Input: part model. Units: mm. Frame: model coordinates. Coordinates: 2 decimals unless noted, no trailing zeros. Loops run counter-clockwise (first coordinate to the right, second up) from the corner with the lowest first, then second, coordinate; pieces in that order, holes last.
(1) Line query: L1, parallel to Z at x = 31.75, y = 3.6; L2, parallel to X at y = 1.65, z = 15; L3, parallel to X at y = 1.8, z = 0. Output: solid intervals per line, ascending.
(2) Section D-D, the plane z = 0. Return loops of the section in (x, y).
(3) Section B-B, the plane x = -31.75. Return loops of the section in (y, z), then the cut area to 4 significant figures.
(4) Section C-C, the plane y = 2.85. Give the number of separate pieces and of enclosed holes in the cut face, then the cut area to 3 significant figures.
(5) Section A-A, the plane z = -15. Return loops of the section in (x, y).
Autodesk Fusion 360 part; units mm, degrees
sketch "Sketch1" plane through (0, 0, 0) normal (0, 1, 0) x (1, 0, 0)
  line L0 (-20.75, -20) -> (20.75, -20) construction
  line L1 (20.75, -20) -> (20.75, 20) construction
  line L2 (20.75, 20) -> (-20.75, 20) construction
  line L3 (-20.75, 20) -> (-20.75, -20) construction
  line L4 (-20.75, -20) -> (20.75, 20) construction
  line L5 (20.75, -20) -> (-20.75, 20) construction
  circle A0 centre (-31.75, 0) radius 4.05
  circle A1 centre (31.75, 0) radius 4.05
  line L6 (25.5, 0) -> (-25.5, 0)
  line L7 (22.803, -2.697) -> (-22.803, -2.697)
  line L8 (-22.803, -2.697) -> (-22.803, -37.303)
  line L9 (-22.803, -37.303) -> (22.803, -37.303)
  line L10 (22.803, -37.303) -> (22.803, -2.697)
  line L11 (22.803, -2.697) -> (-22.803, -37.303) construction
  line L12 (-22.803, -2.697) -> (22.803, -37.303) construction
  line L13 (22.803, 2.697) -> (-22.803, 2.697)
  line L14 (-22.803, 2.697) -> (-22.803, 37.303)
  line L15 (-22.803, 37.303) -> (22.803, 37.303)
  line L16 (22.803, 37.303) -> (22.803, 2.697)
  line L17 (22.803, 2.697) -> (-22.803, 37.303) construction
  line L18 (-22.803, 2.697) -> (22.803, 37.303) construction
  circle A2 centre (-22.803, -37.303) radius 1.55
  circle A3 centre (22.803, -2.697) radius 1.55
  circle A4 centre (-22.803, 2.697) radius 1.55
  circle A5 centre (22.803, 37.303) radius 1.55
  circle A6 centre (-31.75, -15) radius 1.55
  circle A7 centre (-31.75, 15) radius 1.55
  circle A8 centre (31.75, -15) radius 1.55
  circle A9 centre (31.75, 15) radius 1.55
  line L19 (-47, -40) -> (47, -40)
  line L20 (47, -40) -> (47, 40)
  line L21 (47, 40) -> (-47, 40)
  line L22 (-47, 40) -> (-47, -40)
  line L23 (-47, -40) -> (47, 40) construction
  line L24 (47, -40) -> (-47, 40) construction
  point P0 (0, -20)
  point P1 (0, 20)
  point P2 (0, -20)
  point P3 (0, 20)
  dimension "d1" = 41.5
  dimension "d2" = 40
  dimension "d3" = 8.1
  dimension "d4" = 8.1
  dimension "d5" = 11
  dimension "d6" = 11
  dimension "d7" = 51
  dimension "d8" = 20
  dimension "d9" = 20
  dimension "d10" = 45.606
  dimension "d11" = 34.606
  dimension "d12" = 45.606
  dimension "d13" = 34.606
  dimension "d14" = 3.1
  dimension "d15" = 3.1
  dimension "d16" = 3.1
  dimension "d17" = 3.1
  dimension "d18" = 3.1
  dimension "d19" = 3.1
  dimension "d20" = 3.1
  dimension "d21" = 3.1
  dimension "d22" = 15
  dimension "d23" = 15
  dimension "d24" = 15
  dimension "d25" = 15
  dimension "d26" = 94
  dimension "d27" = 80
extrude "Extrude1" add sketch "Sketch1" along normal blind 5 contours L7 L8 L9 L10 A2 A3 | L13 L14 L15 L16 A4 A5 | L19 L20 L21 L22
fillet "Fillet1" radius 10 4 edges at (47, 2.5, 40) (47, 2.5, -40) (-47, 2.5, 40) (-47, 2.5, -40)
equation "d6 = d5"
equation "d23 = d22"
equation "d24 = d23"
equation "d25 = d22"
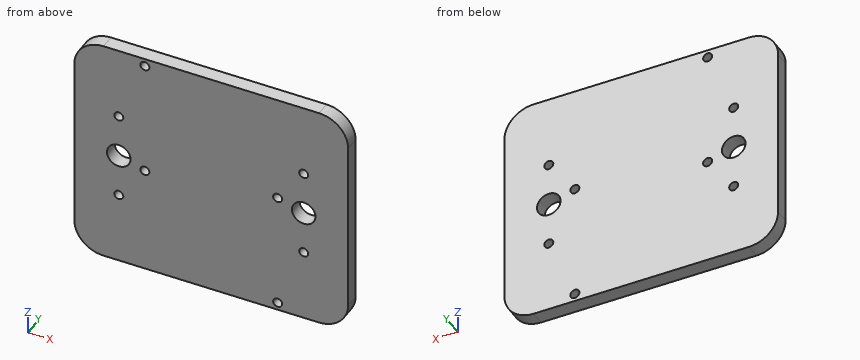
Report:
1. L1: z = -40 to -16.55, -13.45 to -4.05, 4.05 to 13.45, 16.55 to 40
1. L2: x = -47 to -33.3, -30.2 to 30.2, 33.3 to 47
1. L3: x = -47 to -35.8, -27.7 to 27.7, 35.8 to 47
2. outline: (-47, 0) - (-35.8, 0) - (-35.8, 5) - (-47, 5) - close; (-27.7, 0) - (27.7, 0) - (27.7, 5) - (-27.7, 5) - close; (35.8, 0) - (47, 0) - (47, 5) - (35.8, 5) - close
3. outline: (0, -40) - (5, -40) - (5, -16.55) - (0, -16.55) - close; (0, -13.45) - (5, -13.45) - (5, -4.05) - (0, -4.05) - close; (0, 4.05) - (5, 4.05) - (5, 13.45) - (0, 13.45) - close; (0, 16.55) - (5, 16.55) - (5, 40) - (0, 40) - close
3. area: 328.5 mm2
4. separate pieces: 1
4. enclosed holes: 10
4. area: 7,270 mm2
5. outline: (-47, 0) - (-33.3, 0) - (-33.3, 5) - (-47, 5) - close; (-30.2, 0) - (30.2, 0) - (30.2, 5) - (-30.2, 5) - close; (33.3, 0) - (47, 0) - (47, 5) - (33.3, 5) - close
